Geometry check sheet. Reference: drawing and pictorial views, mm from the part's lowest x, y, z. Give positions to 0.01 mm unless a question says otherwise; leave off trailing zeros. Write each loop counter-clockwise with the first axis right and the second up, starting at its lowest first coordinate (ties: lowest second). Pieces come first, ordered by that corner, then holes. Notation, with made-up numbers: M -31,54.25 L 19,54.25 A17 ccw 19,83.25 Z; hole C -25,51 d2. An arc over 180 degrees is marked long. Answer as a JSON object with one key per item and string values.
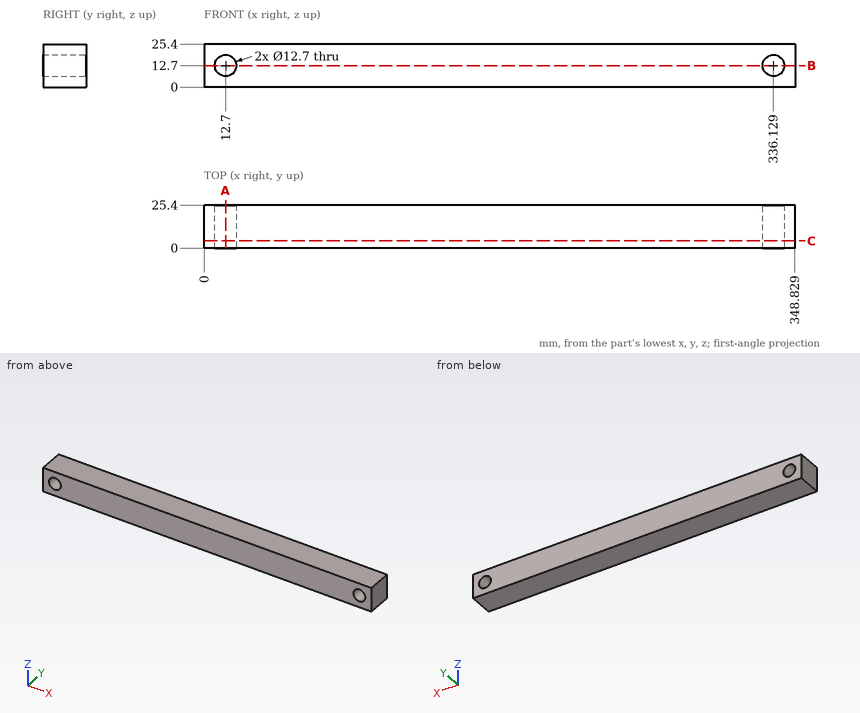
1) Section check B-B on z = 12.7. Record the boundary of the cut face in (x, y).
Completed:
{"outline": "M 0,0 L 6.35,0 L 6.35,25.4 L 0,25.4 Z; M 19.05,0 L 329.78,0 L 329.78,25.4 L 19.05,25.4 Z; M 342.48,0 L 348.83,0 L 348.83,25.4 L 342.48,25.4 Z"}
2) Section check C-C on y = 4.25. Record the boundary of the cut face in (x, z).
Completed:
{"outline": "M 0,0 L 348.83,0 L 348.83,25.4 L 0,25.4 Z; hole C 12.7,12.7 d12.7; hole C 336.13,12.7 d12.7"}
3) Section check A-A on x = 12.7. Record the boundary of the cut face in (y, z), and give its area (3 significant figures).
Completed:
{"outline": "M 0,0 L 25.4,0 L 25.4,6.35 L 0,6.35 Z; M 0,19.05 L 25.4,19.05 L 25.4,25.4 L 0,25.4 Z", "area": "323 mm2"}
4) Go/stop test with a flat-tipped pin: pin 1 (4 mm diameter, centred on x = 276.5, z = 22.5, fed in from -Y). Record where the tip stops, or that it passes through.
Completed:
{"pin 1": "stops at y = 0"}
5) Thickness scan on L1, parallel to X at y = 14.5, z = 13.5; L2, parallel to X at y = 18, z = 12.7; L3, parallel to Z at x = 12.7, y = 9.75. Record the ranges inside material, lowest first.
Completed:
{"L1": "x = 0 to 6.4, 19 to 329.83, 342.43 to 348.83", "L2": "x = 0 to 6.35, 19.05 to 329.78, 342.48 to 348.83", "L3": "z = 0 to 6.35, 19.05 to 25.4"}
